The model under review builds one solid part; all positions refer to its coordinate system, in mm. A direction names the side the tool comes from. Coordinates: 2 decimals unless noted, no trailing zeros. Write each loop counter-clockwise with the first axis right and the second up, starting at its lowest first coordinate (ties: lowest second). Pieces come first, ordered by that corner, then holes. Notation, with made-up numbers: (89, 50) - (101, 50) arc R32 ccw to (101, 87) - close; hole circle Ø9 at (4.25, 26). An arc over 180 degrees is marked (long way). Use one line per item in the form item = value. Start each with the question number.
```python
from build123d import *

# Parameters (mm, degrees)
F0_R     = 9
F1_DEPTH = 35
F4_DEPTH = 25
F5_W     = 10
F5_H     = 6
F6_DEPTH = 5
F7_R     = 1.2910039075
F8_DEPTH = 25


with BuildPart() as f1:
    # F0 (on Front) → F1 (new body)
    with BuildSketch(Plane.XZ):
        Circle(F0_R)
    extrude(amount=F1_DEPTH)

    # F3 (on offset) → F4 (cut)
    with BuildSketch(Plane.XZ.offset(30)):
        with BuildLine():
            ThreePointArc((-7, 0), (0, 7), (7, 0))
            Line((7, 0), (10, 0))
            Line((10, 0), (10, 10))
            Line((10, 10), (-10, 10))
            Line((-10, 10), (-10, 0))
            Line((-10, 0), (-7, 0))
        make_face()
        with BuildLine():
            ThreePointArc((-7, 0), (0, -7), (7, 0))
            Line((7, 0), (-7, 0))
        make_face()
        with BuildLine():
            Line((-7, 0), (7, 0))
            ThreePointArc((7, 0), (0, 7), (-7, 0))
        make_face()
    extrude(amount=-F4_DEPTH, mode=Mode.SUBTRACT)

    # F5 (on face) → F6 (join)
    with BuildSketch(Plane.XZ.offset(35)):
        Rectangle(F5_W, F5_H)
    extrude(amount=F6_DEPTH)

    # F7 (on face) → F8 (cut)
    with BuildSketch(Plane.XY.offset(3)):
        with Locations((0, -36.3444052637)):
            Circle(F7_R)
    extrude(amount=-F8_DEPTH, mode=Mode.SUBTRACT)


solid = f1.part
```
1. The part is to be moulded in two halves that separate along Y. For faces 1 (the flat face through (0, -30, 1)), 2 (the flat face through (0, -38, 3)), 3 (the flat face through (0, -40, 0)), say which applies: released by +Y, released by -Y, zero draft, split by the parting line, or undercut.
2. Take a section at A-A (x = 0). State the section outline as (y, z) points.
3. Take a section at C-C (x = 4.25). State the section outline as (y, z) points.
4. Take a section at B-B (z = 3.5). State the section outline as (x, y) points.
5. Take a section at D-D (y = -33.5). State the section outline as (x, z) points.
6. For L1, parallel to Y at x = 0, z = -1.2; L2, parallel to Y at x = 1.25, z = 3.75; L3, parallel to Y at x = -4.25, z = -0.75, list the stretches that pass through material, from the lowest coordinate up.
7. For P1, Ø2, axis at x = -8, y = -15, coming from the +Z side; P2, Ø1.5, axis at y = -38, z = 1.5, coming from the -X side; P3, Ø1.5, axis at y = -17.5, z = -1.5, coming from the +X side; P4, Ø1.5, axis at x = 0, y = -36.34, coming from the -Z side, all flat-tipped, find the tip position at first contact; note any pin that passes through.
8. For faces 4 (the cylindrical face through (0, -18, -7)), 5 (the flat face through (5, -37, 0)), 6 (the flat face through (-5, -37, 0)), 7 (the flat face through (0, -38, -3)), 8 (the flat face through (-8, -18, 0)), list the 3-axis set-ups (+Z, -Z, +X, -X, +Y, -Y) from which the entire face can be reached by the end or side of a thin tool; tool diameter is ignored.
Returned:
q1.face_1 = undercut
q1.face_2 = zero draft
q1.face_3 = released by -Y
q2.outline = (-40, -3) - (-37.64, -3) - (-37.64, 3) - (-40, 3) - close; (-35.05, -3) - (-35, -3) - (-35, -9) - (0, -9) - (0, 9) - (-5, 9) - (-5, -7) - (-30, -7) - (-30, 9) - (-35, 9) - (-35, 3) - (-35.05, 3) - close
q3.outline = (-40, -3) - (-35, -3) - (-35, -7.93) - (0, -7.93) - (0, 7.93) - (-5, 7.93) - (-5, -5.56) - (-30, -5.56) - (-30, 7.93) - (-35, 7.93) - (-35, 3) - (-40, 3) - close
q4.outline = (-8.29, -35) - (8.29, -35) - (8.29, -30) - (-8.29, -30) - close; (-8.29, -5) - (8.29, -5) - (8.29, 0) - (-8.29, 0) - close
q5.outline = circle Ø18 at (0, 0)
q6.L1 = -40 to -37.64, -35.05 to -30, -5 to 0
q6.L2 = -35 to -30, -5 to 0
q6.L3 = -40 to -30, -5 to 0
q7.P1 = 0
q7.P2 = -5
q7.P3 = 8.97
q7.P4 = through
q8.face_4 = +Z
q8.face_5 = +Z, -Z, +X, -Y
q8.face_6 = +Z, -Z, -X, -Y
q8.face_7 = -Z, +X, -X, -Y
q8.face_8 = +Z, +X, -X
